Source: CAD feature listing. Evaluate the final solid. Frame: model axes, mm. Face numbers are marked on the shaded views. Give positions to 0.01 mm unless a question says otherwise; leave off trailing zeros. Write each loop counter-clockwise with the first axis right and the second up, starting at its lowest first coordinate (ties: lowest second). Pieces come first, ordered by that corner, then holes. Notation, with made-up numbers: (17, 28) - (35, 28) arc R18 cw to (35, 46) - close; hole circle Ø7 at (14, -32). An arc over 180 degrees is marked (long way). Answer as a JSON object with one key per item and string values. Group by question number.
from build123d import *


with BuildPart() as part:
    # Sketch1 → Revolve1 (revolve)
    with BuildSketch(Plane(origin=(0, 0, 0), x_dir=(0, 0, -1), z_dir=(1, 0, 0))):
        with BuildLine():
            Line((5, 2.65), (5, 7.85))
            ThreePointArc((5, 7.85), (4.956066017, 7.956066017), (4.85, 8))
            Line((4.85, 8), (0.15, 8))
            ThreePointArc((0.15, 8), (0.043933983, 7.956066017), (0, 7.85))
            Line((0, 7.85), (0, 2.65))
            ThreePointArc((0, 2.65), (0.043933983, 2.543933983), (0.15, 2.5))
            Line((0.15, 2.5), (4.85, 2.5))
            ThreePointArc((4.85, 2.5), (4.956066017, 2.543933983), (5, 2.65))
        make_face()
    revolve(axis=Axis((0, 0, 0), (0, 0, 1)))


solid = part.part
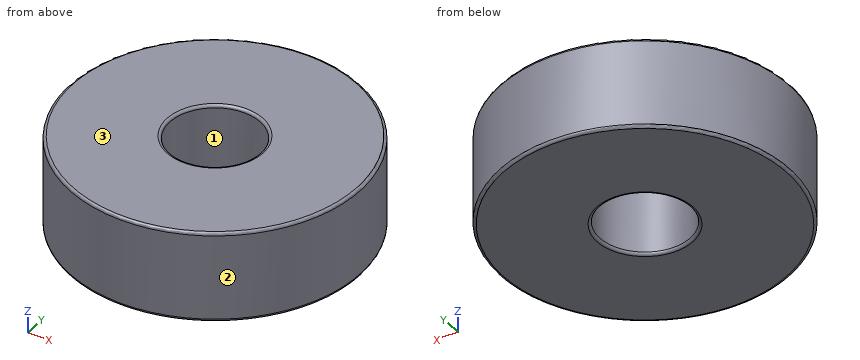
Q1. Draft query along Y for the marked faces 1, 2 and 3. Return one class per face: released by +Y, released by -Y, zero draft, split by the parting line, or undercut.
Q2. First-contact query: pin 1 Ø2 at (x, z) = (-4, -1) entering from +Y; pin 2 Ø1 at (y, z) = (6, -1) entering from +X; pin 3 Ø1.5 at (x, z) = (3.5, -2) entering from +Y; pin 4 Ø4.5 at (x, y) = (0, 0) entering from +Z. Flat tips, straight axial feed; report the tip coordinate or a pass-through.
Q3. Section C-C on z = -0.5. Return the cut outline in (x, y), then the cut area to 3 significant figures.
Q4. Section A-A on x = 0. Return the cut outline in (y, z), then the cut area to 3 significant figures.
Q5. Ray query, probe 1 along X at (y, z) = (0, -3.7); probe 2 along Y at (x, z) = (1, -1.4). Return the intervals inside material, ascending. Write a range as [from, to].
Taken from the geometry:
{
 "1": {"face 1": "undercut", "face 2": "split by the parting line", "face 3": "zero draft"},
 "2": {"pin 1": "stops at y = 7.42", "pin 2": "stops at x = 5.81", "pin 3": "stops at y = 7.51", "pin 4": "passes through"},
 "3": {"outline": "circle Ø16 at (0, 0); hole circle Ø5 at (0, 0)", "area": "181 mm²"},
 "4": {"outline": "(-8, -4.85) arc R0.15 ccw to (-7.85, -5) - (-2.65, -5) arc R0.15 ccw to (-2.5, -4.85) - (-2.5, -0.15) arc R0.15 ccw to (-2.65, 0) - (-7.85, 0) arc R0.15 ccw to (-8, -0.15) - close; (2.5, -4.85) arc R0.15 ccw to (2.65, -5) - (7.85, -5) arc R0.15 ccw to (8, -4.85) - (8, -0.15) arc R0.15 ccw to (7.85, 0) - (2.65, 0) arc R0.15 ccw to (2.5, -0.15) - close", "area": "55.0 mm²"},
 "5": {"probe 1": "x = [-8, -2.5], [2.5, 8]", "probe 2": "y = [-7.94, -2.29], [2.29, 7.94]"}
}
